Check sheet for the modelled part. Datum: model origin and axes. Units: mm. A direction names the side the tool comes from. Round coordinates to 2 decimals unless told otherwise and drop trailing zeros. Write each loop counter-clockwise with the first axis right and the second up, starting at its lowest first coordinate (ties: lowest second). Pieces come first, ordered by that corner, then holes. Notation, with made-up numbers: (-7, 59) - (19, 59) arc R21 cw to (19, 70) - close; hole circle Ø2 at (69.25, 87.5). An arc over 180 degrees is marked (long way). Use one line per item in the form item = value. Start each with the question number.
1) Gauge pin test, flat end, axial feed: P1, Ø1.5, axis at x = -0.5, z = 11, coming from the +Y side. Record the tip position at first contact, or that the pin passes through.
2) Section check B-B (x = 0.65). Record the boundary of the cut face in (y, z), then the cut area to 3 significant figures.
3) Section check A-A (y = 0.25). Record the boundary of the cut face in (x, z), then the cut area to 3 significant figures.
4) Draft check along Z on faces 4 (the face through (0, 0, 10)), 5 (the face through (0, -1, 12)), 6 (the face through (0, 0, 0)), 7 (the face through (0, -5, 6)). Enter one of: +Z half, -Z half, draft (parallel to the pull), parting line (faces both ways), or undercut.
5) Section check C-C (y = 3). Record the boundary of the cut face in (x, z).
6) Set-up check for faces 1 (the face through (0, -0.8, 7)), 2 (the face through (0.02, 0.85, 9.51)), 3 (the face through (0, 2, 5)): record each of +Z, -Z, +X, -X, +Y, -Y from which the full face is reachable in a straight line by a thin tool's end or side.
7) Section check D-D (z = 7). Record the boundary of the cut face in (x, y).
8) Scan lines: probe 1 along Z at (x, y) = (-0.85, -0.5); probe 2 along Z at (x, y) = (-1.1, 3); probe 3 along Y at (x, z) = (0.25, 8). Record each from-to range of solid material in increasing order.
from build123d import *

# Parameters (mm, degrees)
F0_W     = 3
F0_H     = 10
F1_DEPTH = 5
F2_W     = 3
F2_H     = 4.2
F3_DEPTH = 7
F4_W     = 3
F4_H     = 2
F5_DEPTH = 4
F7_DEPTH = 1


with BuildPart() as f1:
    # F0 (on Top) → F1 (new body)
    with BuildSketch(Plane.XY):
        Rectangle(F0_W, F0_H)
    extrude(amount=F1_DEPTH)

    # F2 (on face) → F3 (join)
    with BuildSketch(Plane.XY.offset(5)):
        with Locations((0, -2.9)):
            Rectangle(F2_W, F2_H)
    extrude(amount=F3_DEPTH)

    # F4 (on face) → F5 (join)
    with BuildSketch(Plane(origin=(0, -0.8, 0), x_dir=(-1, 0, 0), z_dir=(0, 1, 0))):
        with Locations((0, 11)):
            Rectangle(F4_W, F4_H)
    extrude(amount=F5_DEPTH)

    # F6 (on face) → F7 (join)
    with BuildSketch(Plane(origin=(0, 0, 10), x_dir=(1, 0, 0), z_dir=(0, 0, -1))):
        Polygon((1.5, -1.069119), (-1.5, -0.6222), (-1.5, -3.2), (1.5, -3.2), align=None)
    extrude(amount=F7_DEPTH)


solid = f1.part
Results are:
q1.P1 = 3.2
q2.outline = (-5, 0) - (5, 0) - (5, 5) - (-0.8, 5) - (-0.8, 10) - (0.94, 10) - (0.94, 9) - (3.2, 9) - (3.2, 12) - (-5, 12) - close
q2.area = 89.7 mm²
q3.outline = (-1.5, 0) - (1.5, 0) - (1.5, 5) - (-1.5, 5) - close; (-1.5, 10) - (1.5, 10) - (1.5, 12) - (-1.5, 12) - close
q3.area = 21.0 mm²
q4.face_4 = undercut
q4.face_5 = +Z half
q4.face_6 = -Z half
q4.face_7 = draft
q5.outline = (-1.5, 0) - (1.5, 0) - (1.5, 5) - (-1.5, 5) - close; (-1.5, 9) - (1.5, 9) - (1.5, 12) - (-1.5, 12) - close
q6.face_1 = +X, -X
q6.face_2 = +X
q6.face_3 = +X, -X, +Y
q7.outline = (-1.5, -5) - (1.5, -5) - (1.5, -0.8) - (-1.5, -0.8) - close
q8.probe_1 = 0 to 5, 10 to 12
q8.probe_2 = 0 to 5, 9 to 12
q8.probe_3 = -5 to -0.8
